Here's how the part is built. I have some questions about the finished solid (model axes, mm). Coordinates: 2 decimals unless noted, no trailing zeros. Loops run counter-clockwise (first coordinate to the right, second up) from the corner with the lowest first, then second, coordinate; pieces in that order, holes last. Notation, with made-up numbers: M 11.5,29.5 L 16.5,29.5 A25 ccw 16.5,43.5 Z; hole C 21.25,76.5 d9. An arc over 180 degrees is marked long. Use one line per item in the form item = value. Start each with the question number.
(1) Please list where these lines run through material, in increasing order: L1, parallel to Y at x = 0, z = 0.75; L2, parallel to X at y = 1.5, z = 0.25; L3, parallel to Y at x = 1, z = 2.3.
(2) Will these pins go through, and if not, where does the flat tip stop? P1, Ø1, axis at y = 2.5, z = 2, coming from the +X side; P2, Ø2, axis at x = -18.5, z = 3, coming from the +Y side.
(3) Imagine slicing it at C-C, the plane z = 2.85. Please give me the cut outline in (x, y).
(4) Imagine slicing it at A-A, the plane x = 0. State how many separate pieces and enclosed holes the cut face has, and give its area (3 significant figures).
(5) Thinking about a two-plate mould opening in Y: for faces 1 (the conical face through (32.26, 1.03, 1.42)), 2 (the cylindrical face through (-8.02, -36.12, 1.98)), 3 (the flat face through (16, -16, 0)), which applies, +Y half, -Y half, draft (parallel to the pull), parting line (faces both ways), or undercut?
```python
from build123d import *

# Parameters (mm, degrees)
F0_R     = 37
F0_R_2   = 3.25
F0_R_3   = 20
F1_DEPTH = 4
F2_SIZE  = 2.75
F3_SIZE  = 0.5


with BuildPart() as f1:
    # F0 (on Top) → F1 (new body)
    with BuildSketch(Plane.XY):
        Circle(F0_R)
        with Locations((0, -29)):
            Circle(F0_R_2, mode=Mode.SUBTRACT)
        with Locations((-29, 0)):
            Circle(F0_R_2, mode=Mode.SUBTRACT)
        Circle(F0_R_3, mode=Mode.SUBTRACT)
        with Locations((29, 0)):
            Circle(F0_R_2, mode=Mode.SUBTRACT)
        with Locations((0, 29)):
            Circle(F0_R_2, mode=Mode.SUBTRACT)
    extrude(amount=F1_DEPTH)

    # F2
    f2_edges = [f1.edges().sort_by_distance(p)[0] for p in [
        (-3.25, -29, 4),
        (-32.25, 0, 4),
        (-3.25, 29, 4),
        (25.75, 0, 4),
    ]]
    chamfer(f2_edges, length=F2_SIZE)

    # F3
    f3_edges = [f1.edges().sort_by_distance(p)[0] for p in [
        (20, 0, 2),
        (-20, 0, 0),
        (-20, 0, 4),
        (37, 0, 2),
        (-37, 0, 0),
        (-37, 0, 4),
        (-3.25, -29, 0),
        (-32.25, 0, 0),
        (25.75, 0, 0),
        (-3.25, 29, 0),
    ]]
    chamfer(f3_edges, length=F3_SIZE)


solid = f1.part
```
Answer:
q1.L1 = -37 to -32.25, -25.75 to -20, 20 to 25.75, 32.25 to 37
q1.L2 = -36.72 to -32.16, -25.84 to -20.19, 20.19 to 25.84, 32.16 to 36.72
q1.L3 = -36.99 to -33.18, -24.82 to -19.97, 19.97 to 24.82, 33.18 to 36.99
q2.P1 = 36.95
q2.P2 = 32.6
q3.outline = C 0,0 d74; hole C -29,0 d9.7; hole C 0,0 d40; hole C 0,-29 d9.7; hole C 0,29 d9.7; hole C 29,0 d9.7
q4.separate_pieces = 4
q4.enclosed_holes = 0
q4.area = 67.4 mm²
q5.face_1 = undercut
q5.face_2 = parting line
q5.face_3 = draft
